Build history of the part. All positions in model axes, mm. Give positions to 0.01 mm unless a question says otherwise; leave off trailing zeros. Loops run counter-clockwise (first coordinate to the right, second up) from the corner with the lowest first, then second, coordinate; pieces in that order, holes last. Notation, with made-up numbers: (-33, -38) -> (-17, -38) arc R31 cw to (-17, -3) -> close; hole circle Ø4 at (-10.75, 69.25). An arc over 180 degrees is marked (long way). Answer as a JSON object with one key per item and string values. Group by question number.
Q1. Wall check: probe 1 along Z at (x, y) = (1546, 116); probe 2 along Z at (x, y) = (162, 119); probe 3 along Y at (x, z) = (318.5, -119). Give the ranges that are in metal, low to high. Write a range as from..to.
Q2. Band-saw the part on A-A, the plane x = 1257.5. Write the cut outline in (y, z), plus the area to 3 significant figures.
Q3. Drop flat-ended pins along their axis: pin 1 (5 mm diameter, centred on x = 1548, z = -144, fed in from -Y); pin 2 (10 mm diameter, centred on y = 170.5, z = -36, fed in from +X). Give the stop position or say it passes through.
Q4. Band-saw the part on B-B, the plane z = -101. Write the cut outline in (x, y).
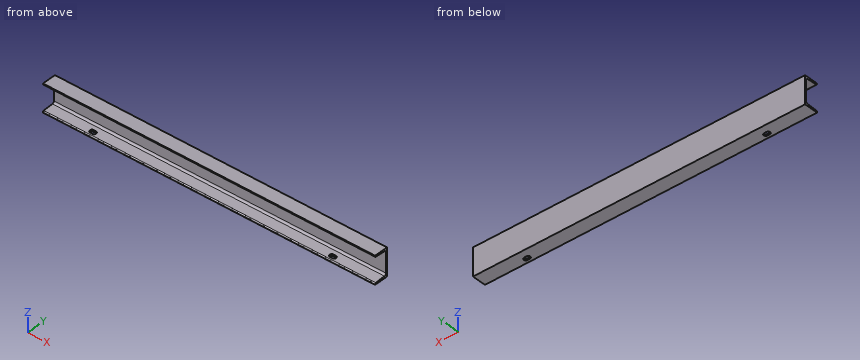
from build123d import *

# Parameters (mm, degrees)
F1_DEPTH = 1800
F3_DEPTH = 9.9223883311


# Not quite as in the source:
# - a pattern or mirror of a feature is missing from the dataset's text; its kind, count and spacing are read off the source's solid


with BuildPart() as f1:
    # F0 (on Right) → F1 (new body)
    with BuildSketch(Plane.YZ):
        with BuildLine():
            Line((185.4237287785, 0), (110.4237287785, 0))
            Line((110.4237287785, 0), (110.4237287785, -3.2898854433))
            ThreePointArc((110.4237287785, -3.2898854433), (111.7968569235, -6.7316583218), (115.1620489973, -8.2830331171))
            Line((115.1620489973, -8.2830331171), (169.447088341, -11.1279914774))
            ThreePointArc((169.447088341, -11.1279914774), (176.1774724886, -14.230741068), (178.9237287785, -21.1142868249))
            Line((178.9237287785, -21.1142868249), (178.9237287785, -128.8857131751))
            ThreePointArc((178.9237287785, -128.8857131751), (176.1774724886, -135.769258932), (169.447088341, -138.8720085226))
            Line((169.447088341, -138.8720085226), (115.1620489973, -141.7169668829))
            ThreePointArc((115.1620489973, -141.7169668829), (111.7968569235, -143.2683416782), (110.4237287785, -146.7101145567))
            Line((110.4237287785, -146.7101145567), (110.4237287785, -150))
            Line((110.4237287785, -150), (185.4237287785, -150))
            Line((185.4237287785, -150), (185.4237287785, 0))
        make_face()
    extrude(amount=F1_DEPTH)

    # F2 (on face) → F3 (cut, through all)
    with BuildSketch(Plane(origin=(0, 0, -150), x_dir=(1, 0, 0), z_dir=(0, 0, -1))):
        with BuildLine():
            ThreePointArc((243.5, -124.4237287785), (232.5, -135.4237287785), (243.5, -146.4237287785))
            Line((243.5, -146.4237287785), (256.5, -146.4237287785))
            ThreePointArc((256.5, -146.4237287785), (267.5, -135.4237287785), (256.5, -124.4237287785))
            Line((256.5, -124.4237287785), (243.5, -124.4237287785))
        make_face()
    f3 = extrude(amount=-F3_DEPTH, mode=Mode.SUBTRACT)

    # F3_copies: F3 across plane
    add(f3.mirror(Plane(origin=(900, 0, 0), x_dir=(0, 0, 1), z_dir=(1, 0, 0))), mode=Mode.SUBTRACT)


solid = f1.part
Worked answers:
{
 "1": {"probe 1": "-150..-141.67, -8.33..0", "probe 2": "-150..-141.52, -8.48..0", "probe 3": "178.92..185.42"},
 "2": {"outline": "(110.42, -150) -> (185.42, -150) -> (185.42, 0) -> (110.42, 0) -> (110.42, -3.29) arc R5 ccw to (115.16, -8.28) -> (169.45, -11.13) arc R10 cw to (178.92, -21.11) -> (178.92, -128.89) arc R10 cw to (169.45, -138.87) -> (115.16, -141.72) arc R5 ccw to (110.42, -146.71) -> close", "area": "2,350 mm2"},
 "3": {"pin 1": "y = 110.43", "pin 2": "through"},
 "4": {"outline": "(0, 178.92) -> (1800, 178.92) -> (1800, 185.42) -> (0, 185.42) -> close"}
}
